Could you check a few things on this drawing? It's one solid part, dimensions in mm from its lowest x, y, z. A direction names the side the tool comes from. Give positions to 0.01 mm unless a question says otherwise; leave off trailing zeros. Order: outer loops, then holes, each group sorted by start corner. A loop starts at its lowest first (then second) coordinate and runs counter-clockwise, first axis right, second up. Notation, with made-up numbers: (-17.75, 76) -> (-0.75, 76) arc R22 cw to (-0.75, 113) -> close; hole circle Ø6 at (73.25, 3). An arc over 180 degrees is marked (long way). Answer as CSV lines item,"result".
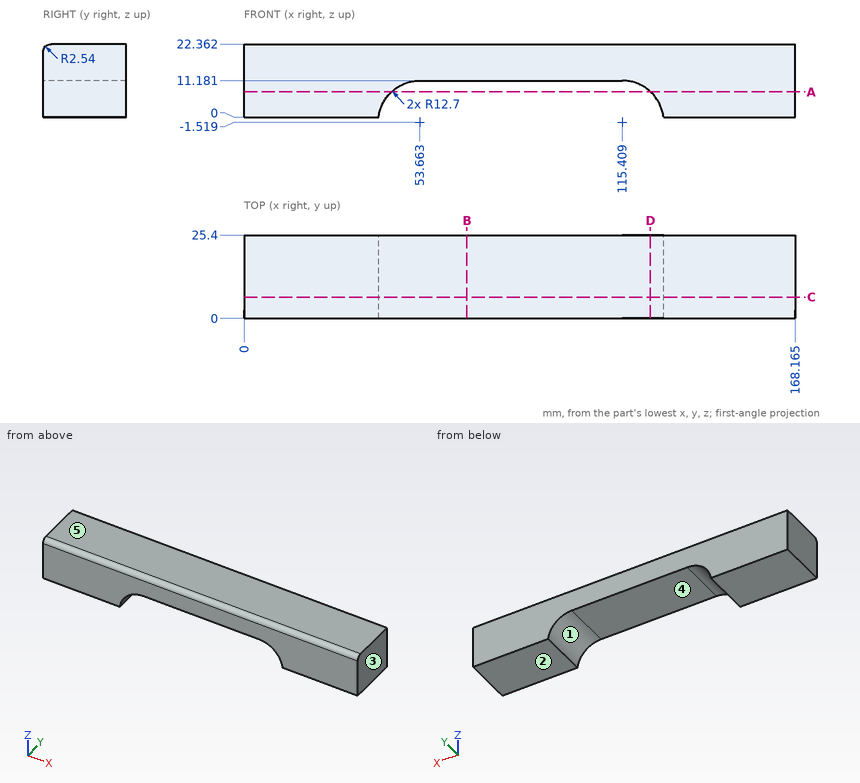
Item 1: Imagine slicing it at B-B, the plane x = 68. Please give me the cut outline in (y, z), then the cut area to 3 significant figures.
Numbers:
outline,"(0, 11.18) -> (25.4, 11.18) -> (25.4, 22.36) -> (2.54, 22.36) arc R2.54 ccw to (0, 19.82) -> close"
area,"283 mm²"
Item 2: We'd pull the mould along X, two halves only. Please class the marked faces 1, 2 and 3: released by +X, released by -X, zero draft, split by the parting line, or undercut.
Numbers:
face 1,"undercut"
face 2,"zero draft"
face 3,"released by +X"
Item 3: Imagine slicing it at C-C, the plane y = 6.5. Please give me the cut outline in (x, z) (1 decimal).
Numbers:
outline,"(0, 0) -> (41.1, 0) arc R12.7 cw to (53.7, 11.2) -> (115.4, 11.2) arc R12.7 cw to (128, 0) -> (168.2, 0) -> (168.2, 22.4) -> (0, 22.4) -> close"
Item 4: For pin 1 (1 mm diameter, centred on x = 124, y = 21.5, fed in from -Z); pin 2 (12.5 mm diameter, centred on x = 85.5, y = 17, fed in from -Z); pin 3 (4 mm diameter, centred on x = 54, y = 8, fed in from -Z), each with a flat end and sliding along its axis, tell me the tip position at first contact or that it passes through.
Numbers:
pin 1,"stops at z = 7.35"
pin 2,"stops at z = 11.18"
pin 3,"stops at z = 11.07"
Item 5: Imagine slicing it at A-A, the plane z = 7.75. Please give me the cut outline in (x, y) (1 decimal).
Numbers:
outline,"(0, 0) -> (45, 0) -> (45, 25.4) -> (0, 25.4) -> close; (124.1, 0) -> (168.2, 0) -> (168.2, 25.4) -> (124.1, 25.4) -> close"
Item 6: Please list where these lines run through material, in increasing order: line 1 along X through (y, z) = (18, 4.5) (1 decimal); line 2 along Z through (x, y) = (63, 8.5); line 3 along X through (y, z) = (13, 2.25) (1 decimal).
Numbers:
line 1,"x = 0 to 42.5, 126.6 to 168.2"
line 2,"z = 11.18 to 22.36"
line 3,"x = 0 to 41.5, 127.5 to 168.2"
Item 7: For the marked faces 4 and 5, which set-ups out of +Z, -Z, +X, -X, +Y, -Y let a thin tool reach every point of the face, with its end or its side?
Numbers:
face 4,"-Z, +Y, -Y"
face 5,"+Z, +X, -X, +Y, -Y"
Item 8: Imagine slicing it at D-D, the plane x = 124. Please give me the cut outline in (y, z) (1 decimal).
Numbers:
outline,"(0, 7.8) -> (25.4, 7.8) -> (25.4, 22.4) -> (2.5, 22.4) arc R2.5 ccw to (0, 19.8) -> close"
